```python
from build123d import *

# Parameters (mm, degrees)
F0_R     = 4.7625
F1_DEPTH = 11.1633
F2_R     = 3.175
F3_DEPTH = 15.8242
F4_R     = 1.35255
F5_DEPTH = 6.35
F6_R     = 1.35255
F7_DEPTH = 6.35


with BuildPart() as f1:
    # F0 (on Top) → F1 (new body)
    with BuildSketch(Plane.XY):
        Circle(F0_R)
    extrude(amount=F1_DEPTH)

    # F2 (on face) → F3 (join)
    with BuildSketch(Plane.XY.offset(11.1633)):
        Circle(F2_R)
    extrude(amount=F3_DEPTH)

    # F4 (on face) → F5 (cut)
    with BuildSketch(Plane(origin=(0, 0, 0), x_dir=(1, 0, 0), z_dir=(0, 0, -1))):
        Circle(F4_R)
    extrude(amount=-F5_DEPTH, mode=Mode.SUBTRACT)

    # F6 (on face) → F7 (cut)
    with BuildSketch(Plane.XY.offset(26.9875)):
        Circle(F6_R)
    extrude(amount=-F7_DEPTH, mode=Mode.SUBTRACT)


solid = f1.part
```
Source: CAD feature listing. Evaluate the final solid. Frame: model axes, mm. A direction names the side the tool comes from. Round coordinates to 2 decimals unless told otherwise and drop trailing zeros. Write each loop counter-clockwise with the first axis right and the second up, starting at its lowest first coordinate (ties: lowest second). Pieces come first, ordered by that corner, then holes. Notation, with made-up numbers: M 7.5,46.5 L 51.5,46.5 A27 ccw 51.5,68.5 Z; hole C 63.5,19 d11. An arc over 180 degrees is marked long. Answer as a JSON object with one key per item and string values. Group by question number.
(1) First-contact query: pin 1 (1.5 mm diameter, centred on y = -1, z = 8, fed in from -X); pin 2 (2 mm diameter, centred on y = 3, z = 23.5, fed in from -X); pin 3 (2 mm diameter, centred on x = 1, z = 22, fed in from -Y) (3 decimals). Flat tips, straight axial feed; report the tip coordinate or a pass-through.
(2) Mould query, pull axis X, two halves, no side actions, for faces 1 (the flat face through (1.4, -0.7, 26.987)), 2 (the cylindrical face through (-3.78, -2.9, 5.5)), 3 (the flat face through (0, 0, 20.638)). Classes: +X half, -X half, draft (parallel to the pull), parting line (faces both ways), or undercut.
(3) Section query C-C on z = 2.75. Output: boundary loops of the cut face in (x, y) (1 decimal).
(4) Ray query, line 1 (Z direction, x = -1, y = 3.5); line 2 (X direction, y = -1.5, z = 14.25); line 3 (X direction, y = 1.25, z = 13.5). Return the intervals inside material, ascending. Write a range as [from, to].
(5) Reachability of faces 4 (the flat face through (0, 0, 6.35)), 5 (the cylindrical face through (1.29, 0.41, 23.86)), 6 (the flat face through (-1.1, 1.1, 0)) from +Z, -Z, +X, -X, +Y, -Y: full face, straight path, thin tool, end or side. Return the list, or none.
(6) Section query D-D on z = 19. Output: boundary loops of the cut face in (x, y) (3 decimals), then the cut area to 3 significant figures.
Computed values:
{
 "1": {"pin 1": "x = -4.76", "pin 2": "x = -2.47", "pin 3": "y = -3.175"},
 "2": {"face 1": "draft", "face 2": "parting line", "face 3": "undercut"},
 "3": {"outline": "C 0,0 d9.5; hole C 0,0 d2.7"},
 "4": {"line 1": "[0, 11.16]", "line 2": "[-2.8, 2.8]", "line 3": "[-2.92, 2.92]"},
 "5": {"face 4": "-Z", "face 5": "+Z", "face 6": "-Z, +X, -X, +Y, -Y"},
 "6": {"outline": "C 0,0 d6.35", "area": "31.7 mm^2"}
}
